Verification items for the finished model (mm, model axes). A direction names the side the tool comes from. Give positions to 0.01 mm unless a question says otherwise; leave off trailing zeros. Write each loop counter-clockwise with the first axis right and the second up, starting at its lowest first coordinate (ties: lowest second). Pieces come first, ordered by that corner, then holes. Notation, with made-up numbers: (-38, -32.5) -> (7, -32.5) arc R28 cw to (7, -5.5) -> close; hole circle Ø3 at (45.5, 62.5). An arc over 180 degrees is marked (long way). Write item = value, one per line.
from build123d import *

# Parameters (mm, degrees)
BASE_FLANGE1_DEPTH      = 15
BASE_FLANGE1_DEPTH_BACK = 15
SKETCH2_R               = 1.5875
CUT_EXTRUDE1_DEPTH      = 72.239034244
SKETCH3_R               = 1.984375
CUT_EXTRUDE2_DEPTH      = 10
FILLET1_R               = 3


# Sheet-metal steps are written as plain solids
with BuildPart() as part:
    # Sketch1 → Base-Flange1 (new, two sides: drawn at the far end of the back side and taken through both)
    with BuildSketch(Plane.XY.offset(-BASE_FLANGE1_DEPTH_BACK)):
        with BuildLine():
            Line((25, 0), (2, 0))
            ThreePointArc((2, 0), (0.585786438, 0.585786438), (0, 2))
            Line((0, 2), (0, 65))
            Line((0, 65), (-0.8, 65))
            Line((-0.8, 65), (-0.8, 2))
            ThreePointArc((-0.8, 2), (0.020101013, 0.020101013), (2, -0.8))
            Line((2, -0.8), (25, -0.8))
            Line((25, -0.8), (25, 0))
        make_face()
    extrude(amount=BASE_FLANGE1_DEPTH + BASE_FLANGE1_DEPTH_BACK)

    # Sketch2 → Cut-Extrude1 (cut, through all)
    with BuildSketch(Plane(origin=(0, 0, 0), x_dir=(0, 0, -1), z_dir=(1, 0, 0))):
        with Locations((0, 55.99)):
            Circle(SKETCH2_R)
    extrude(amount=-CUT_EXTRUDE1_DEPTH, mode=Mode.SUBTRACT)

    # Sketch3 → Cut-Extrude2 (cut)
    with BuildSketch(Plane(origin=(0, 0, 0), x_dir=(1, 0, 0), z_dir=(0, 1, 0))):
        with Locations(Location((15, -5, 0), (0, 0, 270))):
            Circle(SKETCH3_R)
        with Locations(Location((15, 5, 0), (0, 0, 270))):
            Circle(SKETCH3_R)
    extrude(amount=-CUT_EXTRUDE2_DEPTH, mode=Mode.SUBTRACT)

    # Fillet1
    fillet1_edges = [part.edges().sort_by_distance(p)[0] for p in [
        (-0.4, 65, 15),
        (-0.4, 65, -15),
    ]]
    fillet(fillet1_edges, radius=FILLET1_R)


solid = part.part
Item 1: Go/stop test with flat-tipped pins: P1, Ø4, axis at y = 55.99, z = 0, coming from the +X side; P2, Ø7, axis at x = 16.5, z = 3, coming from the +Y side. Record where each tip stops, or that it passes through.
Response values:
P1 = 0
P2 = 0
Item 2: Set-up check for faces 4 (the flat face through (0, 33, 0)), 5 (the flat face through (-0.4, 30.7, -15)): record each of +Z, -Z, +X, -X, +Y, -Y from which the full face is reachable in a straight line by a thin tool's end or side.
Response values:
face_4 = +Z, -Z, +X, +Y
face_5 = -Z, +X, -X, +Y, -Y
Item 3: Sectioned sample at C-C on z = 5. Record the cut outline in (x, y).
Response values:
outline = (-0.8, 2) arc R2.8 ccw to (2, -0.8) -> (13.02, -0.8) -> (13.02, 0) -> (2, 0) arc R2 cw to (0, 2) -> (0, 65) -> (-0.8, 65) -> close; (16.98, -0.8) -> (25, -0.8) -> (25, 0) -> (16.98, 0) -> close
Item 4: Sectioned sample at B-B on x = 15. Record the cut outline in (y, z).
Response values:
outline = (-0.8, -15) -> (0, -15) -> (0, -6.98) -> (-0.8, -6.98) -> close; (-0.8, -3.02) -> (0, -3.02) -> (0, 3.02) -> (-0.8, 3.02) -> close; (-0.8, 6.98) -> (0, 6.98) -> (0, 15) -> (-0.8, 15) -> close
Item 5: Material ranges on line 1 (X direction, y = 13, z = 12.25); line 2 (X direction, y = -0.3, z = -5), recorded low to high.
Response values:
line_1 = -0.8 to 0
line_2 = 0.4 to 13.02, 16.98 to 25
Item 6: Sectioned sample at A-A on y = 55.99. Record the cut outline in (x, z).
Response values:
outline = (-0.8, -15) -> (0, -15) -> (0, -1.59) -> (-0.8, -1.59) -> close; (-0.8, 1.59) -> (0, 1.59) -> (0, 15) -> (-0.8, 15) -> close
Item 7: Sectioned sample at D-D on z = -8. Record the cut outline in (x, y).
Response values:
outline = (-0.8, 2) arc R2.8 ccw to (2, -0.8) -> (25, -0.8) -> (25, 0) -> (2, 0) arc R2 cw to (0, 2) -> (0, 65) -> (-0.8, 65) -> close
Item 8: Mould release check, pull along X, two halves, no side actions. Record for faces 1 (the cylindrical face through (-0.41, 64.1, 14.14)), 2 (the flat face through (-0.8, 34, 0)), 3 (the cylindrical face through (13.063, -0.394, 4.57)): +X half, -X half, draft (parallel to the pull), parting line (faces both ways), or undercut.
Response values:
face_1 = draft
face_2 = -X half
face_3 = undercut
